from build123d import *

# Parameters (mm, degrees)
BOSS_EXTRUDE2_DEPTH = 1.27
SKETCH2_R           = 3.175
BOSS_EXTRUDE4_DEPTH = 3.81


with BuildPart() as part:
    # Sketch1 → Boss-Extrude2 (new body)
    with BuildSketch(Plane.XY):
        with BuildLine():
            Line((-10.19943336, 0), (-10.19943336, 12.7))
            Line((-10.19943336, 12.7), (1.22933034, 26.320270199))
            ThreePointArc((1.22933034, 26.320270199), (2.50056664, 26.913057421), (3.77180294, 26.320270199))
            Line((3.77180294, 26.320270199), (15.20056664, 12.7))
            Line((15.20056664, 12.7), (15.20056664, 0))
            Line((15.20056664, 0), (-10.19943336, 0))
        make_face()
    extrude(amount=BOSS_EXTRUDE2_DEPTH)

    # Sketch2 → Boss-Extrude4 (add)
    with BuildSketch(Plane.XY.offset(1.27)):
        with Locations(Location((2.50056664, 19.293057421, 0), (0, 0, 180))):
            Circle(SKETCH2_R)
    extrude(amount=BOSS_EXTRUDE4_DEPTH)


solid = part.part
The listing builds one solid part. Answer for the finished solid, in the listing's coordinates (mm). A direction names the side the tool comes from. Round coordinates to 2 decimals unless told otherwise and drop trailing zeros. Order: outer loops, then holes, each group sorted by start corner. A loop starts at its lowest first (then second) coordinate and runs counter-clockwise, first axis right, second up. Notation, with made-up numbers: M 55,-19.5 L 71,-19.5 A18 cw 71,8.5 Z; hole C 55,-34.75 d3. An arc over 180 degrees is marked long. Answer in a Markdown table with one row per item. Add a question column.
1) Consider line 1 along Z through (x, y) = (10, 10.75); line 2 along Y through (x, z) = (5.25, 3.55); line 3 along Y through (x, z) = (-1, 1.1). Determine where each line is inside the solid, lowest interval first. Write a range as from..to.
2) The part is cut by section D-D on y = 5. Determine the outline of the cut face in (x, z).
3) Which of the six approach directions +Z, -Z, +X, -X, +Y, -Y give full straight-line access (tool end or side, diameter ignored) to faces 1 (the face through (9.406, 19.605, 0.626)), 2 (the face through (2.914, 16.145, 3.148))?
4) The part is cut by section B-B on y = 18.25. Determine the outline of the cut face in (x, z).
5) The part is cut by section C-C on x = 4.75. Determine the outline of the cut face in (y, z).
6) The part is cut by section A-A on z = 0.65. Determine the outline of the cut face in (x, y), plus the area to 3 significant figures.
7) A flat-ended cylindrical pin translates along its axis: pin 1 Ø1 at (x, z) = (-3, 1.5) entering from +Y. Find the tip coordinate at first contact, or state that the pin passes through.
Findings below:
| question | item | result |
|---|---|---|
| 1 | line 1 | z = 0..1.27 |
| 1 | line 2 | y = 17.71..20.88 |
| 1 | line 3 | y = 0..23.66 |
| 2 | outline | M -10.2,0 L 15.2,0 L 15.2,1.27 L -10.2,1.27 Z |
| 3 | face 1 | +Z, -Z, +X, +Y |
| 3 | face 2 | +Z |
| 4 | outline | M -5.54,0 L 10.54,0 L 10.54,1.27 L 5.5,1.27 L 5.5,5.08 L -0.5,5.08 L -0.5,1.27 L -5.54,1.27 Z |
| 5 | outline | M 0,0 L 25.15,0 L 25.15,1.27 L 21.53,1.27 L 21.53,5.08 L 17.05,5.08 L 17.05,1.27 L 0,1.27 Z |
| 6 | outline | M -10.2,0 L 15.2,0 L 15.2,12.7 L 3.77,26.32 A1.66 ccw 1.23,26.32 L -10.2,12.7 Z |
| 6 | area | 514 mm² |
| 7 | pin 1 | stops at y = 21.81 |
